```python
from build123d import *

# Parameters (mm, degrees)
SKETCH1_W           = 300
SKETCH1_H           = 210
SKETCH1_W_2         = 148
SKETCH1_H_2         = 150
BOSS_EXTRUDE1_DEPTH = 1.5
SKETCH2_W           = 62
SKETCH2_H           = 68
SKETCH2_R           = 5
BOSS_EXTRUDE2_DEPTH = 3


with BuildPart() as part:
    # Sketch1 → Boss-Extrude1 (new, symmetric)
    with BuildSketch(Plane(origin=(0, 0, 0), x_dir=(1, 0, 0), z_dir=(0, 1, 0))):
        Rectangle(SKETCH1_W, SKETCH1_H)
        Rectangle(SKETCH1_W_2, SKETCH1_H_2, mode=Mode.SUBTRACT)
    extrude(amount=BOSS_EXTRUDE1_DEPTH, both=True)

    # Sketch2 → Boss-Extrude2 (add, through all)
    with BuildSketch(Plane(origin=(0, 1.5, 0), x_dir=(1, 0, 0), z_dir=(0, 1, 0))):
        with Locations((0, 139)):
            Rectangle(SKETCH2_W, SKETCH2_H)
        with Locations(Location((0, 138, 0), (0, 0, 270))):
            Circle(SKETCH2_R, mode=Mode.SUBTRACT)
    extrude(amount=-BOSS_EXTRUDE2_DEPTH)


solid = part.part
```
Part model, mm, in its own coordinate system. Round coordinates to 2 decimals unless told otherwise and drop trailing zeros. Write each loop counter-clockwise with the first axis right and the second up, starting at its lowest first coordinate (ties: lowest second). Pieces come first, ordered by that corner, then holes. Notation, with made-up numbers: M 6.5,-15.75 L 51.5,-15.75 A12 ccw 51.5,4.25 Z; hole C 41,-19.75 d1. An arc over 180 degrees is marked long. One line per question, with ' | ' between items.
(1) Saw through at B-B on x = 0. Write the cut outline in (y, z), then the cut area to 3 significant figures.
Answer key:
outline: M -1.5,-173 L 1.5,-173 L 1.5,-143 L -1.5,-143 Z; M -1.5,-133 L 1.5,-133 L 1.5,-75 L -1.5,-75 Z; M -1.5,75 L 1.5,75 L 1.5,105 L -1.5,105 Z | area: 354 mm^2
(2) Probe line 1 along X through (y, z) = (0.35, -138); line 2 along X through (y, z) = (-0.9, 61.5); line 3 along Z through (x, y) = (-56, -0.7). List the from-to ranges inside material, lowest first.
Answer key:
line 1: x = -31 to -5, 5 to 31 | line 2: x = -150 to -74, 74 to 150 | line 3: z = -105 to -75, 75 to 105
(3) Pin check, flat tips, straight feed: pin 1 (1.5 mm diameter, centred on x = -109.5, y = -0.5, fed in from -Z); pin 2 (1.5 mm diameter, centred on y = -0.5, z = -126.5, fed in from -X); pin 3 (1.5 mm diameter, centred on y = -0.5, z = -122, fed in from +X). Stop position of each tip, or through.
Answer key:
pin 1: stops at z = -105 | pin 2: stops at x = -31 | pin 3: stops at x = 31
(4) Saw through at C-C on y = -0.2. Write the cut outline in (x, z).
Answer key:
outline: M -150,-105 L -31,-105 L -31,-173 L 31,-173 L 31,-105 L 150,-105 L 150,105 L -150,105 Z; hole M -74,-75 L 74,-75 L 74,75 L -74,75 Z; hole C 0,-138 d10
(5) Saw through at A-A on z = -38. Write the cut outline in (x, y), then the cut area to 3 significant figures.
Answer key:
outline: M -150,-1.5 L -74,-1.5 L -74,1.5 L -150,1.5 Z; M 74,-1.5 L 150,-1.5 L 150,1.5 L 74,1.5 Z | area: 456 mm^2
(6) Saw through at D-D on x = -62. Write the cut outline in (y, z).
Answer key:
outline: M -1.5,-105 L 1.5,-105 L 1.5,-75 L -1.5,-75 Z; M -1.5,75 L 1.5,75 L 1.5,105 L -1.5,105 Z
(7) Two-plate mould, pull along X, no slides. Class faces 1 (the face through (-3, 0, -142)), 2 (the face through (-2, 1.5, -98)): released by +X, released by -X, zero draft, split by the parting line, or undercut.
Answer key:
face 1: undercut | face 2: zero draft
